Design review of the part built by this model. Coordinates are the model's own, in mm. A direction names the side the tool comes from. Give positions to 0.01 mm unless a question says otherwise; leave off trailing zeros. Order: outer loops, then holes, each group sorted by start corner. A loop starts at its lowest first (then second) coordinate and runs counter-clockwise, first axis right, second up. Notation, with made-up numbers: (70, 65.25) -> (96, 65.25) arc R24 ccw to (96, 89.25) -> close; hole circle Ø3 at (4.25, 39.25). An arc over 180 degrees is marked (long way). Use a Markdown table: item, result. Add a question column.
```python
from build123d import *

# Parameters (mm, degrees)
F0_W     = 600
F0_H     = 2496
F1_DEPTH = 1200
F2_W     = 1200
F2_H     = 96
F3_DEPTH = 10
F4_W     = 1100
F4_H     = 160
F5_DEPTH = 580


with BuildPart() as f1:
    # F0 (on Right) → F1 (new body)
    with BuildSketch(Plane.YZ):
        Rectangle(F0_W, F0_H)
    extrude(amount=F1_DEPTH)

    # F2 (on face) → F3 (cut)
    with BuildSketch(Plane.XZ.offset(300)):
        with Locations((600, -1200)):
            Rectangle(F2_W, F2_H)
    extrude(amount=-F3_DEPTH, mode=Mode.SUBTRACT)

    # F4 (on face) → F5 (cut)
    with BuildSketch(Plane.XZ.offset(300)):
        with Locations((600, -1052)):
            Rectangle(F4_W, F4_H)
    extrude(amount=-F5_DEPTH, mode=Mode.SUBTRACT)


solid = f1.part
```
1) For L1, parallel to Z at x = 906.5, y = 100.5; L2, parallel to X at y = -213, z = -972.5, list the stretches that pass through material, from the lowest coordinate up. Write a range as [from, to].
2) The part is to be moulded in two halves that separate along X. For faces 1 (the flat face through (1200, -4, 17)), 2 (the flat face through (592, -290, -1199)), 3 (the flat face through (0, -4, 17)), 4 (the flat face through (1150, -14, -1053)), say which applies: +X half, -X half, draft (parallel to the pull), parting line (faces both ways), or undercut.
3) Add section A-A (x = 341). Give the boundary of the cut face in (y, z), then the cut area to 3 significant figures.
4) Machinability: for faces 5 (the flat face through (592, 300, -17)), 6 (the flat face through (592, -14, -972)), which of the approach directions +Z, -Z, +X, -X, +Y, -Y give a long, thin tool a straight path to every point of the face, cutting with its end or side? Answer none if there is none.
5) Insertion check: pin 1 (8 mm diameter, centred on x = 531, y = -293.5, fed in from -Z). The pin has a flat end and moves straight along its axis. Give the tip position at first contact, or say it passes through.
6) Add section B-B (y = -228). Give the boundary of the cut face in (x, z).
Worked answers:
| question | item | result |
|---|---|---|
| 1 | L1 | [-1248, -1132], [-972, 1248] |
| 1 | L2 | [0, 50], [1150, 1200] |
| 2 | face 1 | +X half |
| 2 | face 2 | draft |
| 2 | face 3 | -X half |
| 2 | face 4 | undercut |
| 3 | outline | (-300, -1152) -> (-290, -1152) -> (-290, -1248) -> (300, -1248) -> (300, 1248) -> (-300, 1248) -> (-300, -972) -> (280, -972) -> (280, -1132) -> (-300, -1132) -> close |
| 3 | area | 1,400,000 mm^2 |
| 4 | face 5 | +Z, -Z, +X, -X, +Y |
| 4 | face 6 | -Y |
| 5 | pin 1 | z = -1248 |
| 6 | outline | (0, -1248) -> (1200, -1248) -> (1200, 1248) -> (0, 1248) -> close; hole (50, -1132) -> (1150, -1132) -> (1150, -972) -> (50, -972) -> close |
